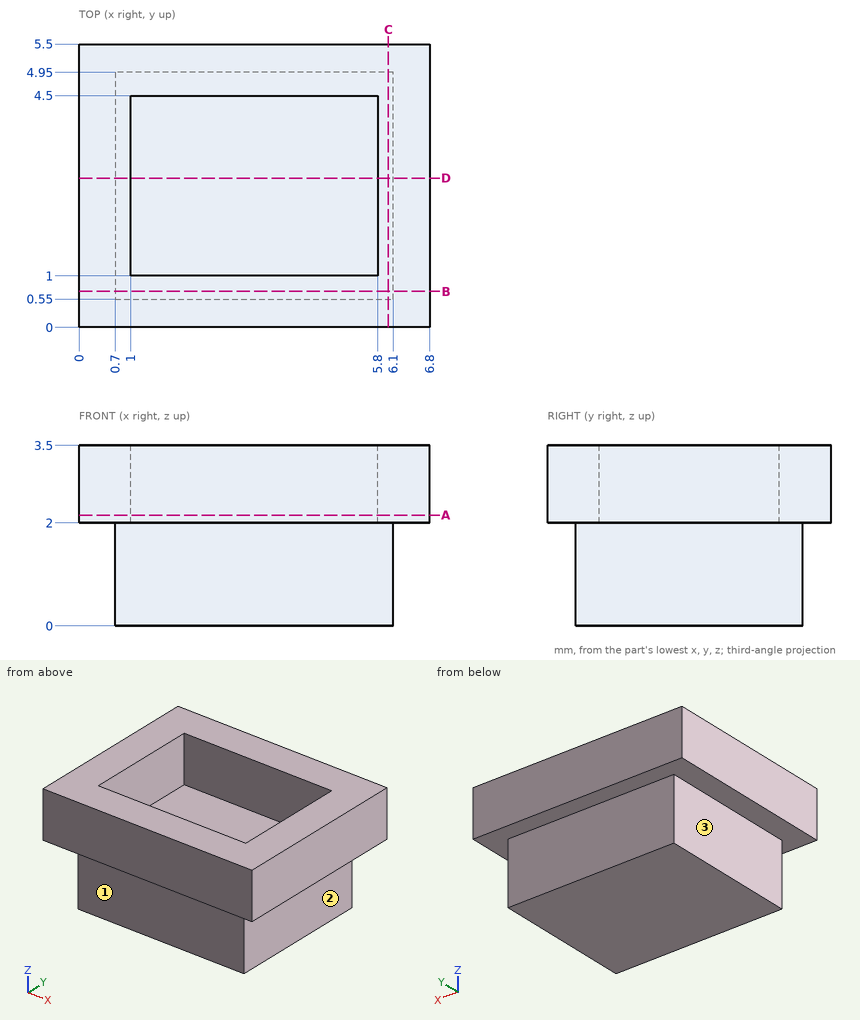
Geometry: see drawing. Coordinates: mm, zero at the bounding-box minimum. A direction names the side the tool comes from. Round coordinates to 2 decimals unless told otherwise and drop trailing zeros. Write each loop counter-clockwise with the first axis right and the second up, starting at its lowest first coordinate (ties: lowest second). Pieces come first, ordered by that corner, then holes. Notation, with made-up numbers: (61.5, -19) -> (105.5, -19) arc R20 ccw to (105.5, -1) -> close; hole circle Ø9 at (-34, -32). An arc over 180 degrees is marked (long way). Answer as CSV lines item,"result".
1. Reachability of the marked faces 1, 2 and 3 from +Z, -Z, +X, -X, +Y, -Y: full face, straight path, thin tool, end or side. Return the list, or none.
Geometry says:
face 1,"-Z, +X, -X, -Y"
face 2,"-Z, +X, +Y, -Y"
face 3,"-Z, -X, +Y, -Y"
2. Section B-B (y = 0.7). Return the cut outline in (x, z), plus the area to 3 significant figures.
Geometry says:
outline,"(0, 2) -> (0.7, 2) -> (0.7, 0) -> (6.1, 0) -> (6.1, 2) -> (6.8, 2) -> (6.8, 3.5) -> (0, 3.5) -> close"
area,"21.0 mm^2"
3. Section C-C (x = 6). Return the cut outline in (y, z), plus the area to 4 significant figures.
Geometry says:
outline,"(0, 2) -> (0.55, 2) -> (0.55, 0) -> (4.95, 0) -> (4.95, 2) -> (5.5, 2) -> (5.5, 3.5) -> (0, 3.5) -> close"
area,"17.05 mm^2"
4. Ray query, L1, parallel to X at y = 1.45, z = 2.55; L2, parallel to Y at x = 4.5, z = 3.05; L3, parallel to Y at x = 5.25, z = 1.65. Return the intervals inside material, ascending. Write a range as [from, to].
Geometry says:
L1,"x = [0, 1], [5.8, 6.8]"
L2,"y = [0, 1], [4.5, 5.5]"
L3,"y = [0.55, 4.95]"
5. Section A-A (z = 2.15). Return the cut outline in (x, y), plus the area to 3 significant figures.
Geometry says:
outline,"(0, 0) -> (6.8, 0) -> (6.8, 5.5) -> (0, 5.5) -> close; hole (1, 1) -> (5.8, 1) -> (5.8, 4.5) -> (1, 4.5) -> close"
area,"20.6 mm^2"
6. Contact query for flat-ended pins moving along their axis: P1, Ø1, axis at x = 4, y = 2.5, coming from the +Z side; P2, Ø1, axis at x = 2.5, z = 1, coming from the -Y side; P3, Ø0.8, axis at x = 3.5, z = 3, coming from the -Y side; P4, Ø1.6, axis at x = 3, z = 1, coming from the +Y side. Output: stop coordinate, or through.
Geometry says:
P1,"stops at z = 2"
P2,"stops at y = 0.55"
P3,"stops at y = 0"
P4,"stops at y = 4.95"
7. Section D-D (y = 2.9). Return the cut outline in (x, z).
Geometry says:
outline,"(0, 2) -> (0.7, 2) -> (0.7, 0) -> (6.1, 0) -> (6.1, 2) -> (6.8, 2) -> (6.8, 3.5) -> (5.8, 3.5) -> (5.8, 2) -> (1, 2) -> (1, 3.5) -> (0, 3.5) -> close"
